```python
from build123d import *

# Parameters (mm, degrees)
F1_DEPTH = 100
F2_DEPTH = 50
F3_W     = 6.8111047149
F3_H     = 3.6732461303
F3_W_2   = 4.2452551425
F3_H_2   = 4.9546863884
F4_DEPTH = 25
F3_H_3   = 3.0913013034
F3_H_4   = 6.5471306443
F5_DEPTH = 100
F6_DEPTH = 5


with BuildPart() as f1:
    # F0 (on Top) → F1 (new body)
    with BuildSketch(Plane.XY):
        with BuildLine():
            ThreePointArc((-56.0795928311, -23.3514428312), (-43.6321915412, -57.9434272798), (-14.1167279775, -36.0258407891))
            ThreePointArc((-14.1167279775, -36.0258407891), (-15.2963829561, -28.7714614887), (-18.7137881744, -22.2646230493))
            ThreePointArc((-18.7137881744, -22.2646230493), (-37.0660364689, -34.1762047765), (-56.0795928311, -23.3514428312))
        make_face()
        with BuildLine():
            ThreePointArc((-56.0795928311, -23.3514428312), (-37.0660364689, -34.1762047765), (-18.7137881744, -22.2646230493))
            ThreePointArc((-18.7137881744, -22.2646230493), (-37.6778941182, -13.1400092827), (-56.0795928311, -23.3514428312))
        make_face()
    extrude(amount=F1_DEPTH)

    # F0 (on Top) → F2 (join)
    with BuildSketch(Plane.XY):
        with BuildLine():
            ThreePointArc((-56.0795928311, -23.3514428312), (-37.6778941182, -13.1400092827), (-18.7137881744, -22.2646230493))
            ThreePointArc((-18.7137881744, -22.2646230493), (-17.1596431946, -17.8194611389), (-16.6328022762, -13.1400092827))
            ThreePointArc((-16.6328022762, -13.1400092827), (-42.9519082998, 7.2335192543), (-56.0795928311, -23.3514428312))
        make_face()
    extrude(amount=F2_DEPTH)

    # F3 (on face) → F4 (join)
    with BuildSketch(Plane.XY.offset(50)):
        with Locations((-34.9110998213, -8.3837537095)):
            Rectangle(F3_W, F3_H)
        with Locations((-45.1333094388, -9.0244738385)):
            Rectangle(F3_W_2, F3_H_2)
    extrude(amount=F4_DEPTH)

    # F3 (on face) → F5 (join)
    with BuildSketch(Plane.XY.offset(50)):
        with Locations((-34.9110998213, -5.0014799926)):
            Rectangle(F3_W, F3_H_3)
        with Locations((-45.1333094388, -3.2735653222)):
            Rectangle(F3_W_2, F3_H_4)
    extrude(amount=F5_DEPTH)

    # F3 (on face) → F6 (join)
    with BuildSketch(Plane.XY.offset(50)):
        Polygon((-31.5055474639, -6.5471306443), (-25.4983492196, -6.5471306443), (-25.4983492196, 2.0140481647), (-49.141228199, 2.0140481647), (-49.141228199, -6.5471306443), (-47.25593701, -6.5471306443), (-47.25593701, 0), (-43.0106818676, 0), (-43.0106818676, -6.5471306443), (-38.3166521788, -6.5471306443), (-38.3166521788, -3.455829341), (-31.5055474639, -3.455829341), align=None)
    extrude(amount=F6_DEPTH)


solid = f1.part
```
The model under review builds one solid part; all positions refer to its coordinate system, in mm. A direction names the side the tool comes from. Round coordinates to 2 decimals unless told otherwise and drop trailing zeros. Loops run counter-clockwise (first coordinate to the right, second up) from the corner with the lowest first, then second, coordinate; pieces in that order, holes last.
1) Consider section D-D on x = -22.5. State the section outline as (y, z) points, then the cut area to 3 significant figures.
Values follow:
outline: (-53.73, 0) - (1.44, 0) - (1.44, 50) - (-18.32, 50) - (-18.32, 100) - (-53.73, 100) - close
area: 4,530 mm2
2) Consider section A-A on z = 109.5. State the section outline as (x, y) points, then the cut area to 3 significant figures.
Values follow:
outline: (-47.26, -6.55) - (-43.01, -6.55) - (-43.01, 0) - (-47.26, 0) - close; (-38.32, -6.55) - (-31.51, -6.55) - (-31.51, -3.46) - (-38.32, -3.46) - close
area: 48.8 mm2
3) Clearance check with flat-ended pins moving along their axes: P1, Ø7, axis at x = -31.5, y = -0.5, coming from the +Z side; P2, Ø3.5, axis at y = -7.5, z = 106.5, coming from the -X side; P3, Ø2, axis at x = -50.5, y = -8, coming from the +Z side; P4, Ø2, axis at x = -44, z = 66.5, coming from the -Y side. State where each tip first meets the part, or that it passes through.
Values follow:
P1: stops at z = 150
P2: stops at x = -47.26
P3: stops at z = 50
P4: stops at y = -58.12
4) Consider section C-C on y = -19. State the section outline as (x, z) points, then the cut area to 3 significant figures.
Values follow:
outline: (-57.89, 0) - (-17.47, 0) - (-17.47, 50) - (-21.7, 50) - (-21.7, 100) - (-52.32, 100) - (-52.32, 50) - (-57.89, 50) - close
area: 3,550 mm2
5) The part is to be moulded in two halves that separate along X. For faces 4 (the face through (-49.141, -2, 52)), 5 (the face through (-41, -6.547, 52)), 6 (the face through (-35, -10.22, 62)), say which applies: pulls with the +X half, pulls with the -X half, needs draft (parallel to the pull), parting line crosses it, or undercut.
Values follow:
face 4: pulls with the -X half
face 5: undercut
face 6: needs draft
6) Wall thickness on line 1 along Z through (x, y) = (-18.5, -37.5); line 2 along Z through (x, y) = (-33, -11); line 3 along Y through (x, z) = (-34, 108): over which ranges is each line inside the solid? List them lowest first.
Values follow:
line 1: z = 0 to 100
line 2: z = 0 to 50
line 3: y = -6.55 to -3.46
7) Consider section B-B on z = 80. State the section outline as (x, y) points, then the cut area to 3 significant figures.
Values follow:
outline: circle Ø45.79 at (-37.01, -36.03); (-47.26, -6.55) - (-43.01, -6.55) - (-43.01, 0) - (-47.26, 0) - close; (-38.32, -6.55) - (-31.51, -6.55) - (-31.51, -3.46) - (-38.32, -3.46) - close
area: 1,700 mm2
8) Tool access review of faces 1 (the face through (-25.498, -2, 52)), 2 (the face through (-37, -36, 100)), 3 (the face through (-45, -9, 75)): name each direction out of +Z, -Z, +X, -X, +Y, -Y from which nothing blocks a thin tool from reaching the whole face with its end or side.
Values follow:
face 1: +Z, +X, +Y
face 2: +Z, +X, -X, -Y
face 3: +Z, +X, -X
